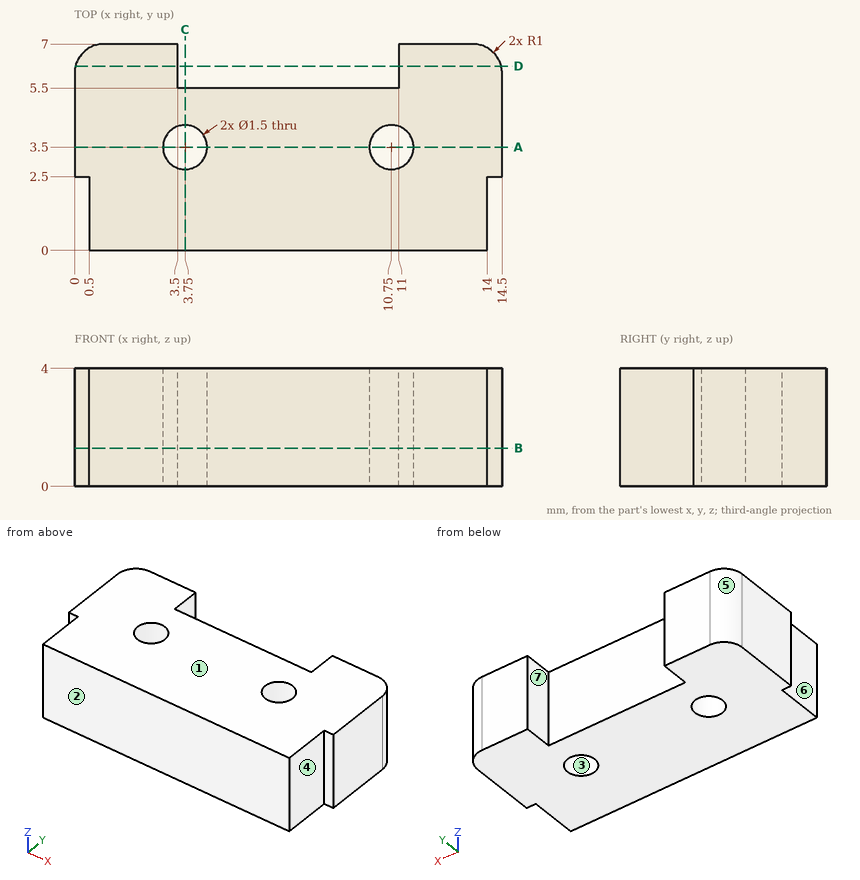
Part print with two shaded views. Sizes in mm from the minimum x, y, z corner. A direction names the side the tool comes from. Coordinates: 2 decimals unless noted, no trailing zeros. Loops run counter-clockwise (first coordinate to the right, second up) from the corner with the lowest first, then second, coordinate; pieces in that order, holes last. Notation, with made-up numbers: M -24,46 L -18,46 A22 ccw -18,83 Z; hole C -22,74.5 d4. An arc over 180 degrees is marked long. Use CSV: the item, a comma, the result in double quotes. Start each with the question number.
1. Band-saw the part on D-D, the plane y = 6.25. List the corners of the cut face in (x, z).
2. Probe probe 1 along Y at (x, z) = (10.75, 2.95); probe 2 along X at (y, z) = (4, 0.2); probe 3 along Y at (x, z) = (8, 2.6). List the from-to ranges inside material, lowest first. Write a range as [from, to].
3. Flat gauge pins, fed straight in: pin 1 (1 mm diameter, centred on x = 9, z = 1, fed in from +Y); pin 2 (0.8 mm diameter, centred on y = 6.5, z = 3, fed in from +X) (3 decimals); pin 3 (1.7 mm diameter, centred on x = 3.75, y = 3.5, fed in from +Z); pin 4 (1.4 mm diameter, centred on x = 10.75, y = 3.5, fed in from +Z). Where does each tip first touch, or does it go through?
4. Band-saw the part on C-C, the plane x = 3.75. List the corners of the cut face in (y, z).
5. Two-plate mould, pull along Y, no slides. Class the marked faces 1, 2 and 3: pulls with the +Y half, pulls with the -Y half, needs draft (parallel to the pull), parting line crosses it, or undercut.
6. Band-saw the part on B-B, the plane z = 1.3. List the corners of the cut face in (x, y), then the cut area to 3 significant figures.
7. Tool access for the marked faces 4, 5, 6 and 7: list every direction of +Z, -Z, +X, -X, +Y, -Y with a clear straight run to the whole face (end or side of a thin tool).
8. Band-saw the part on A-A, the plane y = 3.5. List the corners of the cut face in (x, z).
Entries:
1,outline,"M 0.03,0 L 3.5,0 L 3.5,4 L 0.03,4 Z; M 11,0 L 14.47,0 L 14.47,4 L 11,4 Z"
2,probe 1,"y = [0, 2.75], [4.25, 5.5]"
2,probe 2,"x = [0, 3.19], [4.31, 10.19], [11.31, 14.5]"
2,probe 3,"y = [0, 5.5]"
3,pin 1,"stops at y = 5.5"
3,pin 2,"stops at x = 14.495"
3,pin 3,"stops at z = 4"
3,pin 4,"passes through"
4,outline,"M 0,0 L 2.75,0 L 2.75,4 L 0,4 Z; M 4.25,0 L 5.5,0 L 5.5,4 L 4.25,4 Z"
5,face 1,"needs draft"
5,face 2,"pulls with the -Y half"
5,face 3,"undercut"
6,outline,"M 0,2.5 L 0.5,2.5 L 0.5,0 L 14,0 L 14,2.5 L 14.5,2.5 L 14.5,6 A1 ccw 13.5,7 L 11,7 L 11,5.5 L 3.5,5.5 L 3.5,7 L 1,7 A1 ccw 0,6 Z; hole C 3.75,3.5 d1.5; hole C 10.75,3.5 d1.5"
6,area,"83.8 mm2"
7,face 4,"+Z, -Z, +X, -Y"
7,face 5,"+Z, -Z, -X, +Y"
7,face 6,"+Z, -Z, -X, -Y"
7,face 7,"+Z, -Z, +Y"
8,outline,"M 0,0 L 3,0 L 3,4 L 0,4 Z; M 4.5,0 L 10,0 L 10,4 L 4.5,4 Z; M 11.5,0 L 14.5,0 L 14.5,4 L 11.5,4 Z"
